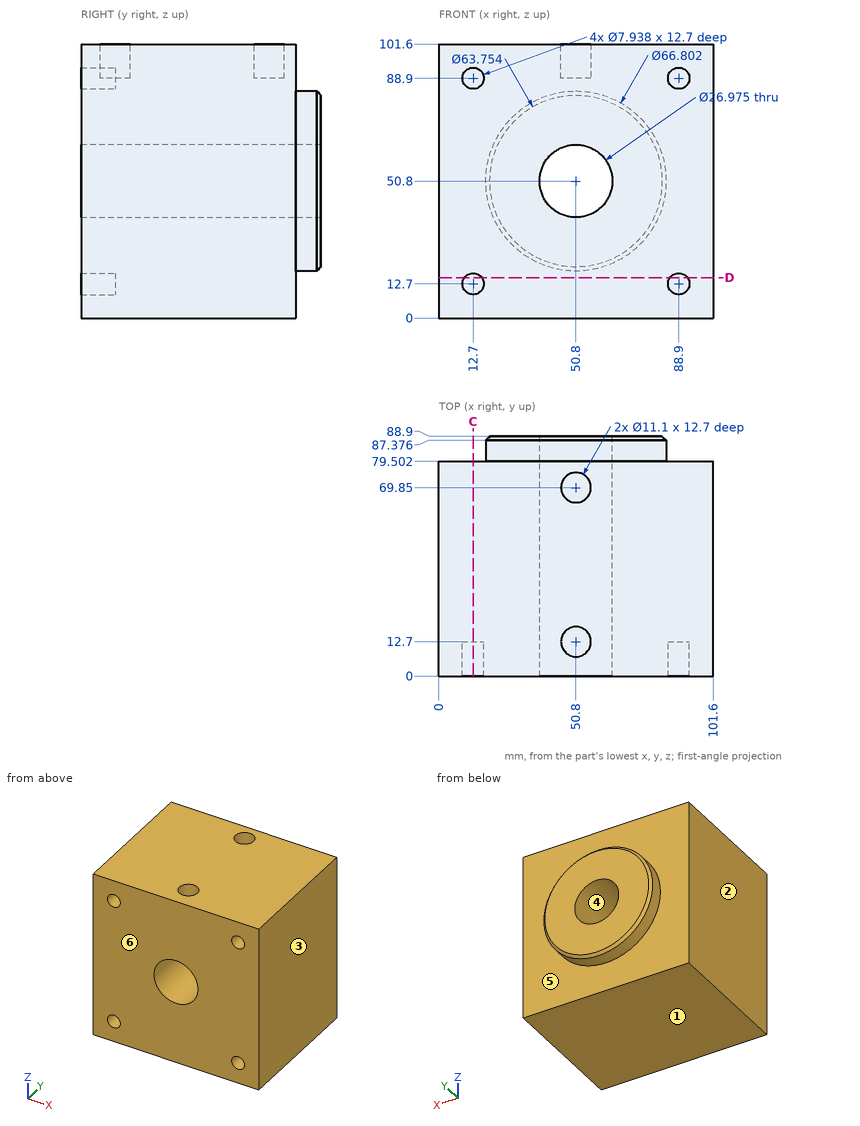
For this review, use the dimensioned drawing (mm, ordinates from the lowest corner) and the shaded views. A direction names the side the tool comes from. Round coordinates to 2 decimals unless told otherwise and drop trailing zeros. Write each loop counter-clockwise with the first axis right and the second up, starting at its lowest first coordinate (ties: lowest second). Pieces come first, ordered by that corner, then holes. Notation, with made-up numbers: M 65.5,72.5 L 88.5,72.5 A16 cw 88.5,80.5 Z; hole C 4,81.25 d3. An arc over 180 degrees is marked long. Use CSV: the item, a comma, the result in double quotes. Start each with the question number.
(1) The part is to be moulded in two halves that separate along X. For the marked faces 1, 2, 3 and 4, say which applies: +X half, -X half, draft (parallel to the pull), parting line (faces both ways), or undercut.
(2) For line 1 along Y through (x, z) = (50.8, 93.5); line 2 along X through (y, z) = (3, 88.9); line 3 along Z through (x, y) = (50, 38), list the stretches that pass through material, from the lowest coordinate up.
(3) We need section C-C, the plane x = 12.7. State the section outline as (y, z) points.
(4) Clearance check with flat-ended pins moving along their axes: P1, Ø4, axis at x = 11, z = 72.5, coming from the +Y side; P2, Ø7, axis at x = 88.9, z = 88.9, coming from the -Y side; P3, Ø5.5, axis at x = 49.5, y = 13.5, coming from the +Z side; P4, Ø16, axis at x = 50.8, z = 50.8, coming from the +Y side. State where each tip first meets the part, or that it passes through.
(5) We need section D-D, the plane z = 15. State the section outline as (x, y) points (1 decimal).
(6) Tool access review of the marked faces 5 and 6: name each direction out of +Z, -Z, +X, -X, +Y, -Y from which nothing blocks a thin tool from reaching the whole face with its end or side.
Findings:
1,face 1,"draft"
1,face 2,"-X half"
1,face 3,"+X half"
1,face 4,"undercut"
2,line 1,"0 to 7.15, 18.25 to 64.3, 75.4 to 79.5"
2,line 2,"0 to 8.73, 16.67 to 84.93, 92.87 to 101.6"
2,line 3,"0 to 37.34, 64.26 to 101.6"
3,outline,"M 0,0 L 79.5,0 L 79.5,101.6 L 0,101.6 L 0,92.87 L 12.7,92.87 L 12.7,84.93 L 0,84.93 L 0,16.67 L 12.7,16.67 L 12.7,8.73 L 0,8.73 Z"
4,P1,"y = 79.5"
4,P2,"y = 12.7"
4,P3,"z = 88.9"
4,P4,"through"
5,outline,"M 0,0 L 9.5,0 L 9.5,12.7 L 15.9,12.7 L 15.9,0 L 85.7,0 L 85.7,12.7 L 92.1,12.7 L 92.1,0 L 101.6,0 L 101.6,79.5 L 0,79.5 Z"
6,face 5,"+Y"
6,face 6,"+Z, -Z, +X, -X, -Y"
